Geometry check sheet. Reference: the model listing, model coordinates, mm. A direction names the side the tool comes from. Round coordinates to 2 decimals unless told otherwise and drop trailing zeros. Order: outer loops, then holes, each group sorted by start corner. A loop starts at its lowest first (then second) coordinate and runs counter-clockwise, first axis right, second up.
(1) Release check for a two-part mould opening along X. For faces 6 (the face through (72.76, 28.26, -37.76)), 7 (the face through (46, 50.8, 1)), 8 (the face through (58, 12.7, 1)) record: +X half, -X half, draft (parallel to the pull), parting line (faces both ways), or undercut.
(2) Sectioned sample at B-B (y = 82). Record the boundary of the cut face in (x, z).
(3) Set-up check for faces 1 (the face through (-1, 88.9, 1)), 2 (the face through (53.81, 1.45, 37.68)), 3 (the face through (52, 28, 39.207)), 4 (the face through (52.442, 49.351, 0.549)), 5 (the face through (53.81, 1.53, -37.76)): record each of +Z, -Z, +X, -X, +Y, -Y from which the full face is reachable in a straight line by a thin tool's end or side.
(4) Sectioned sample at A-A (y = 70). Record the boundary of the cut face in (x, z) (3 decimals), plus the area to 3 significant figures.
(5) Material ranges on line 1 along X through (y, z) = (40.5, 0) (3 decimals); line 2 along Z through (x, y) = (0, 36) (3 decimals); line 3 along Z through (x, y) = (4, 56.5), recorded low to high.
(6) Go/stop test with flat-tipped pins: pin 1 (12 mm diameter, centred on x = -4.5, y = 49.5, fed in from +Z); pin 2 (25 mm diameter, centred on x = -14.5, z = 5.5, fed in from -Y); pin 3 (1 mm diameter, centred on x = 29, y = 67.5, fed in from +Z). Record where each tip stops, or that it passes through.
from build123d import *

# Parameters (mm, degrees)
F1_DEPTH    = 50.8
F0_W        = 12.7
F0_H        = 78.4147009254
F0_W_2      = 7.62
F2_DEPTH    = 12.7
F3_DEPTH    = 88.9
F5_DEPTH    = 88.9
F7_T1_DEPTH = 50.8
F8_R        = 5.08
F9_R        = 2.54
F11_R       = 44.45
F12_DEPTH   = 8.89


# Not quite as in the source:
# - a fillet or chamfer that OpenCascade refuses, or shapes differently, is made with other operations: its cross-section is extruded or revolved along the edge and cut away or added


with BuildPart() as f1:
    # F0 (on Front) → F1 (new body)
    with BuildSketch(Plane.XZ):
        with BuildLine():
            ThreePointArc((41.2700087631, 16.5102657972), (43.6477627692, 8.4068606055), (44.45, 0))
            ThreePointArc((44.45, 0), (43.6477627692, -8.4068606055), (41.2700087631, -16.5102657972))
            Line((41.2700087631, -16.5102657972), (41.2700087631, -39.2073504627))
            Line((41.2700087631, -39.2073504627), (53.9700087631, -39.2073504627))
            Line((53.9700087631, -39.2073504627), (53.9700087631, 39.2073504627))
            Line((53.9700087631, 39.2073504627), (41.2700087631, 39.2073504627))
            Line((41.2700087631, 39.2073504627), (41.2700087631, 16.5102657972))
        make_face()
    extrude(amount=-F1_DEPTH)



with BuildPart() as f1b:
    # F0 (on Front) → F1, piece 2 (new body)
    with BuildSketch(Plane.XZ):
        with Locations((67.9400087631, 0)):
            Rectangle(F0_W, F0_H)
    extrude(amount=-F1_DEPTH)


with BuildPart() as f1_1:
    add(f1.part)

    add(f1b.part)  # F2 merges F1b
    # F0 (on Front) → F2 (join)
    with BuildSketch(Plane.XZ):
        with Locations((57.7800087631, 0)):
            Rectangle(F0_W_2, F0_H)
    extrude(amount=-F2_DEPTH)

    # F0 (on Front) → F3 (join)
    with BuildSketch(Plane.XZ):
        with BuildLine():
            Line((41.2700087631, 0.6418735824), (41.2700087631, 16.5102657972))
            ThreePointArc((41.2700087631, 16.5102657972), (-44.45, 0), (41.2700087631, -16.5102657972))
            Line((41.2700087631, -16.5102657972), (41.2700087631, -0.6418735824))
            ThreePointArc((41.2700087631, -0.6418735824), (-41.275, 0), (41.2700087631, 0.6418735824))
        make_face()
    extrude(amount=-F3_DEPTH)

    # F4: union 

    # F0 (on Front) → F5 (join)
    with BuildSketch(Plane.XZ):
        with BuildLine():
            ThreePointArc((41.2700087631, -16.5102657972), (43.6477627692, -8.4068606055), (44.45, 0))
            ThreePointArc((44.45, 0), (43.6477627692, 8.4068606055), (41.2700087631, 16.5102657972))
            Line((41.2700087631, 16.5102657972), (41.2700087631, 0.6418735824))
            ThreePointArc((41.2700087631, 0.6418735824), (41.2737521719, 0.3209464941), (41.275, 0))
            ThreePointArc((41.275, 0), (41.2737521719, -0.3209464941), (41.2700087631, -0.6418735824))
            Line((41.2700087631, -0.6418735824), (41.2700087631, -16.5102657972))
        make_face()
    extrude(amount=-F5_DEPTH)

    # F6: union 

    # F7: fillet of radius 7.62 on 2 edges, made by hand

    # F7_s2 → F7_t1 (join)
    with BuildSketch(Plane.XZ.offset(-50.8)):
        with BuildLine():
            ThreePointArc((41.2700087631, -39.2073504627), (36.6353958241, -32.7032366386), (28.7404382359, -33.9085492171))
            ThreePointArc((28.7404382359, -33.9085492171), (36.0699423168, -25.9761768022), (41.2700087631, -16.5102657972))
            Line((41.2700087631, -16.5102657972), (41.2700087631, -39.2073504627))
        make_face()
        with BuildLine():
            ThreePointArc((28.7404382359, 33.9085492171), (36.6353958241, 32.7032366386), (41.2700087631, 39.2073504627))
            Line((41.2700087631, 39.2073504627), (41.2700087631, 16.5102657972))
            ThreePointArc((41.2700087631, 16.5102657972), (36.0699423168, 25.9761768022), (28.7404382359, 33.9085492171))
        make_face()
    extrude(amount=F7_T1_DEPTH)

    # F8
    f8_edges = [f1_1.edges().sort_by_distance(p)[0] for p in [
        (53.970009, 50.8, 0),
        (61.590009, 50.8, 0),
        (74.290009, 0, 0),
        (57.780009, 0, -39.20735),
        (57.780009, 0, 39.20735),
        (74.290009, 50.8, 0),
        (74.290009, 25.4, -39.20735),
        (74.290009, 25.4, 39.20735),
    ]]
    fillet(f8_edges, radius=F8_R)

    # F9
    f9_edges = [f1_1.edges().sort_by_distance(p)[0] for p in [
        (-41.270009, 0, -0.641874),
    ]]
    fillet(f9_edges, radius=F9_R)

    # F11 (on offset) → F12 (join)
    with BuildSketch(Plane(origin=(0, 88.9, 0), x_dir=(-1, 0, 0), z_dir=(0, 1, 0))):
        Circle(F11_R)
    extrude(amount=-F12_DEPTH)


solid = f1_1.part
Answer below:
1. face 6: +X half
1. face 7: draft
1. face 8: undercut
2. outline: circle Ø88.9 at (0, 0)
3. face 1: +Z, -Z, +X, -X, +Y
3. face 2: +Z, +X, -Y
3. face 3: +Z, +X, +Y, -Y
3. face 4: +Z, -Z, +Y
3. face 5: -Z, +X, -Y
4. outline: circle Ø88.9 at (0, 0); hole circle Ø82.55 at (0, 0)
4. area: 855 mm2
5. line 1: x = -44.45 to -41.275, 41.275 to 53.97, 61.59 to 74.29
5. line 2: z = -44.45 to -41.275, 41.275 to 44.45
5. line 3: z = -44.27 to -41.08, 41.08 to 44.27
6. pin 1: stops at z = 44.45
6. pin 2: stops at y = 80.01
6. pin 3: stops at z = 34.11
